Design review of the part built by this model. Coordinates are the model's own, in mm. A direction names the side the tool comes from. Coordinates: 2 decimals unless noted, no trailing zeros. Loops run counter-clockwise (first coordinate to the right, second up) from the corner with the lowest first, then second, coordinate; pieces in that order, holes last. Notation, with made-up numbers: M 50.5,7 L 59.5,7 A15 cw 59.5,15 Z; hole C 78,21 d4. An arc over 180 degrees is marked long. Answer as a JSON object with one key per item and string values. Group by question number.
1. Consider section A-A (x = 42.5). State the section outline as (y, z) points.
2. Insertion check: pin 1 (12 mm diameter, centred on x = 73, y = 4.5, fed in from -Z); pin 2 (4 mm diameter, centred on x = 73, z = -6, fed in from +Y); pin 3 (19 mm diameter, centred on x = 76, y = 0.5, fed in from +Z); pin 4 (25 mm diameter, centred on x = -6.5, y = 10.5, fed in from -Z). Each pin has a flat end and moves straight along its axis. Give the tip position at first contact, or say it passes through.
3. Machinability: for faces 4 (the flat face through (94.7, 10, 9.8)), 5 (the flat face through (44.4, -14, -0.4)), 6 (the flat face through (68, 0, -14)), 7 (the flat face through (94.7, -10, -9.8)), 8 (the flat face through (94.7, 9.8, -10)), which of the approach directions +Z, -Z, +X, -X, +Y, -Y give a long, thin tool a straight path to every point of the face, cutting with its end or side? Answer none if there is none.
4. Consider section B-B (x = 7). State the section outline as (y, z) points, then the cut area to 3 significant figures.
5. Consider section C-C (z = 15.5). State the section outline as (x, y) points.
6. To check wall thickness, follow probe 1 along Y at (x, z) = (0, 24.5); probe 2 along Z at (x, y) = (-9, 11.5); probe 3 along X at (y, z) = (0, -20). State the ranges of each line that lie inside material, in increasing order.
7. Consider section D-D (x = 94). State the section outline as (y, z) points.
8. Draft analysis for pull direction Y (two halves, no side actions). For faces 1 (the cylindrical face through (79.48, -10.66, 10.55)), 2 (the flat face through (113, 0, 0)), 3 (the cylindrical face through (11.923, 3.755, -23.126)), state which applies: +Y half, -Y half, draft (parallel to the pull), parting line (faces both ways), or undercut.
from build123d import *

# Parameters (mm, degrees)
CROQUIS1_R              = 12.5
SALIENTE_EXTRUIR2_DEPTH = 32
CROQUIS3_W              = 110
CROQUIS3_H              = 28
CORTAR_EXTRUIR1_DEPTH   = 32
SALIENTE_EXTRUIR3_DEPTH = 28
CROQUIS9_W              = 30
CROQUIS9_H              = 28
SALIENTE_EXTRUIR4_DEPTH = 14
SALIENTE_EXTRUIR5_DEPTH = 36
REDONDEO2_R             = 5.7


with BuildPart() as part:
    # Croquis1 → Saliente-Extruir2 (new, symmetric)
    with BuildSketch(Plane.XY):
        with BuildLine():
            Line((20.712315177, -14), (30, -14))
            Line((30, -14), (30, 14))
            Line((30, 14), (20.712315177, 14))
            ThreePointArc((20.712315177, 14), (-25, 0), (20.712315177, -14))
        make_face()
        Circle(CROQUIS1_R, mode=Mode.SUBTRACT)
    extrude(amount=SALIENTE_EXTRUIR2_DEPTH, both=True)

    # Croquis3 → Cortar-Extruir1 (cut, symmetric)
    with BuildSketch(Plane(origin=(0, 0, 0), x_dir=(1, 0, 0), z_dir=(0, 1, 0))):
        with Locations((-25, 0)):
            Rectangle(CROQUIS3_W, CROQUIS3_H)
    extrude(amount=CORTAR_EXTRUIR1_DEPTH, both=True, mode=Mode.SUBTRACT)


with BuildPart() as cortar_extruir1_piece_1:
    # of the separate pieces the step leaves, piece 1, a body of its own (cortar_extruir1_pieces)
    add(part.part.solids().sort_by_distance((20.712315177, -14, -14))[0])



with BuildPart() as cortar_extruir1_piece_2:
    # of the separate pieces the step leaves, piece 2, a body of its own (cortar_extruir1_pieces)
    add(part.part.solids().sort_by_distance((20.712315177, -14, 32))[0])


with BuildPart() as cortar_extruir1_piece_1_1:
    add(cortar_extruir1_piece_1.part)

    add(cortar_extruir1_piece_2.part)  # Saliente-Extruir3 merges Cortar-Extruir1 piece 2
    # Croquis7 → Saliente-Extruir3 (add)
    with BuildSketch(Plane(origin=(0, 14, 0), x_dir=(1, 0, 0), z_dir=(0, 1, 0))):
        with BuildLine():
            Line((30, 32), (30, 14))
            ThreePointArc((30, 14), (44, 0), (30, -14))
            Line((30, -14), (30, -32))
            ThreePointArc((30, -32), (62, 0), (30, 32))
        make_face()
    extrude(amount=-SALIENTE_EXTRUIR3_DEPTH)

    # Croquis9 → Saliente-Extruir4 (add, symmetric)
    with BuildSketch(Plane(origin=(0, 0, 0), x_dir=(1, 0, 0), z_dir=(0, 1, 0))):
        with Locations((62, 0)):
            Rectangle(CROQUIS9_W, CROQUIS9_H)
    extrude(amount=SALIENTE_EXTRUIR4_DEPTH, both=True)

    # Croquis10 → Saliente-Extruir5 (add)
    with BuildSketch(Plane(origin=(77, 0, 0), x_dir=(0, 0, -1), z_dir=(1, 0, 0))):
        Polygon((-14.00015584, 5.798613627), (-13.99984415, -5.799366115), (-5.798613627, -14.00015584), (5.799366115, -13.99984415), (14.00015584, -5.798613627), (13.99984415, 5.799366115), (5.798613627, 14.00015584), (-5.799366115, 13.99984415), align=None)
    extrude(amount=SALIENTE_EXTRUIR5_DEPTH)

    # Redondeo2
    redondeo2_edges = [cortar_extruir1_piece_1_1.edges().sort_by_distance(p)[0] for p in [
        (77, -9.899683057, 9.899306813),
        (77, -9.899306813, -9.899683057),
        (77, 9.899683057, -9.899306813),
        (77, 9.899306813, 9.899683057),
    ]]
    fillet(redondeo2_edges, radius=REDONDEO2_R)


solid = cortar_extruir1_piece_1_1.part
Findings below:
{
 "1": {"outline": "M -14,-29.46 L 14,-29.46 L 14,-6.3 L -14,-6.3 Z; M -14,6.3 L 14,6.3 L 14,29.46 L -14,29.46 Z"},
 "2": {"pin 1": "stops at z = -14", "pin 2": "stops at y = 14", "pin 3": "stops at z = 14", "pin 4": "stops at z = -32"},
 "3": {"face 4": "+Z, +X, +Y", "face 5": "+Z, -Z, +X, -Y", "face 6": "-Z, +X, +Y, -Y", "face 7": "-Z, +X, -Y", "face 8": "-Z, +X, +Y"},
 "4": {"outline": "M -24,-32 L -10.36,-32 L -10.36,-14 L -24,-14 Z; M -24,14 L -10.36,14 L -10.36,32 L -24,32 Z; M 10.36,-32 L 24,-32 L 24,-14 L 10.36,-14 Z; M 10.36,14 L 24,14 L 24,32 L 10.36,32 Z", "area": "982 mm^2"},
 "5": {"outline": "M 20.71,-14 L 58,-14 L 58,14 L 20.71,14 A25 ccw long Z; hole C 0,0 d25"},
 "6": {"probe 1": "y = -25 to -12.5, 12.5 to 25", "probe 2": "z = -32 to -14, 14 to 32", "probe 3": "x = -25 to -12.5, 12.5 to 54.98"},
 "7": {"outline": "M -14,-5.8 L -5.8,-14 L 5.8,-14 L 14,-5.8 L 14,5.8 L 5.8,14 L -5.8,14 L -14,5.8 Z"},
 "8": {"face 1": "-Y half", "face 2": "draft", "face 3": "undercut"}
}
